The model under review builds one solid part; all positions refer to its coordinate system, in mm. A direction names the side the tool comes from. Coordinates: 2 decimals unless noted, no trailing zeros. Loops run counter-clockwise (first coordinate to the right, second up) from the corner with the lowest first, then second, coordinate; pieces in that order, holes last. Notation, with made-up numbers: M 78.25,16 L 108.25,16 A26 ccw 108.25,37 Z; hole C 0.25,84 d6. An arc over 180 degrees is marked long. Use one line per item in the form item = value.
```python
from build123d import *

# Parameters (mm, degrees)
ESQUISSE1_W             = 21.59
ESQUISSE1_H             = 12.7
ESQUISSE1_W_2           = 15.24
ESQUISSE1_H_2           = 6.35
BOSS_EXTRU_1_DEPTH      = 596.9
ESQUISSE2_R             = 4.7244
ESQUISSE2_W             = 6.858
ESQUISSE2_H             = 6.35
ENL_V_MAT_EXTRU_1_DEPTH = 598.132675396
ESQUISSE3_W             = 63.5
ESQUISSE3_H             = 21.59
ENL_V_MAT_EXTRU_2_DEPTH = 598.132675396


with BuildPart() as part:
    # Esquisse1 → Boss.-Extru.1 (new body)
    with BuildSketch(Plane(origin=(0, 0, 0), x_dir=(0, 0, -1), z_dir=(1, 0, 0))):
        Rectangle(ESQUISSE1_W, ESQUISSE1_H)
        Rectangle(ESQUISSE1_W_2, ESQUISSE1_H_2, mode=Mode.SUBTRACT)
    extrude(amount=BOSS_EXTRU_1_DEPTH)

    # Esquisse2 → Enlèv. mat.-Extru.1 (cut, through all)
    with BuildSketch(Plane.XZ.offset(6.35)):
        with Locations(Location((31.75, 0, 0), (0, 0, 270))):
            Circle(ESQUISSE2_R)
        with Locations((9.525, 0)):
            Rectangle(ESQUISSE2_W, ESQUISSE2_H)
        with Locations((53.975, 0)):
            Rectangle(ESQUISSE2_W, ESQUISSE2_H)
    enl_v_mat_extru_1 = extrude(amount=-ENL_V_MAT_EXTRU_1_DEPTH, mode=Mode.SUBTRACT)

    # Symétrie1: Enlèv. mat.-Extru.1 across plane
    add(enl_v_mat_extru_1.mirror(Plane.ZY.offset(-298.45)), mode=Mode.SUBTRACT)

    # Esquisse3 → Enlèv. mat.-Extru.2 (cut, through all)
    with BuildSketch(Plane.XZ.offset(6.35)):
        with Locations((565.15, 0)):
            Rectangle(ESQUISSE3_W, ESQUISSE3_H)
    extrude(amount=-ENL_V_MAT_EXTRU_2_DEPTH, mode=Mode.SUBTRACT)


solid = part.part
```
1. Insertion check: P1, Ø5.5, axis at x = 31.75, z = 0, coming from the -Y side. The pin has a flat end and moves straight along its axis. Give the tip position at first contact, or say it passes through.
Response values:
P1 = through
2. The part is to be moulded in two halves that separate along Y. For faces 1 (the face through (263, 3.175, 0)), 2 (the face through (263, -6.35, 0)), 3 (the face through (263, 0, 10.795)), say which applies: pulls with the +Y half, pulls with the -Y half, needs draft (parallel to the pull), parting line crosses it, or undercut.
Response values:
face_1 = undercut
face_2 = pulls with the -Y half
face_3 = needs draft
3. Wall thickness on line 1 along X through (y, z) = (-4.5, 1); line 2 along X through (y, z) = (5.1, 0); line 3 along Y through (x, z) = (71.5, -5.5) (3 decimals): over which ranges is each line inside the solid? List them lowest first. Write a range as from..to.
Response values:
line_1 = 0..6.1, 12.95..27.13, 36.37..50.55, 57.4..533.4
line_2 = 0..6.1, 12.95..27.03, 36.47..50.55, 57.4..533.4
line_3 = -6.35..-3.175, 3.175..6.35
4. Add section A-A (x = 326.5). State the section outline as (y, z) points (3 decimals).
Response values:
outline = M -6.35,-10.795 L 6.35,-10.795 L 6.35,10.795 L -6.35,10.795 Z; hole M -3.175,-7.62 L 3.175,-7.62 L 3.175,7.62 L -3.175,7.62 Z
5. Add section C-C (x = 31.75). State the section outline as (y, z) points (3 decimals), then the cut area to 3 significant figures.
Response values:
outline = M -6.35,-10.795 L 6.35,-10.795 L 6.35,-4.724 L 3.175,-4.724 L 3.175,-7.62 L -3.175,-7.62 L -3.175,-4.724 L -6.35,-4.724 Z; M -6.35,4.724 L -3.175,4.724 L -3.175,7.62 L 3.175,7.62 L 3.175,4.724 L 6.35,4.724 L 6.35,10.795 L -6.35,10.795 Z
area = 117 mm^2
6. Add section B-B (y = 1). State the section outline as (x, z) points (3 decimals), then the cut area to 3 significant figures.
Response values:
outline = M 0,-10.795 L 533.4,-10.795 L 533.4,-7.62 L 0,-7.62 Z; M 0,7.62 L 533.4,7.62 L 533.4,10.795 L 0,10.795 Z
area = 3,390 mm^2
7. Machinability: for faces 4 (the face through (263, -3.175, 0)), 5 (the face through (263, 0, -10.795)), which of the approach directions +Z, -Z, +X, -X, +Y, -Y give a long, thin tool a straight path to every point of the face, cutting with its end or side? Answer none if there is none.
Response values:
face_4 = +X, -X
face_5 = -Z, +X, -X, +Y, -Y
